from build123d import *

# Parameters (mm, degrees)
SKETCH3_R = 4
P_L_DEPTH = 10


with BuildPart() as part:
    # Sketch1 → Revolve1 (revolve)
    with BuildSketch(Plane.XY):
        with BuildLine():
            Line((-25, 2), (14.8, 2))
            Line((14.8, 2), (15, 1.946410162))
            Line((15, 1.946410162), (15, 1.85))
            ThreePointArc((15, 1.85), (15.029289322, 1.779289322), (15.1, 1.75))
            Line((15.1, 1.75), (15.208578644, 1.75))
            ThreePointArc((15.208578644, 1.75), (15.246846987, 1.757612047), (15.279289322, 1.779289322))
            Line((15.279289322, 1.779289322), (15.5, 2))
            Line((15.5, 2), (26.5, 2))
            Line((26.5, 2), (27, 1.5))
            Line((27, 1.5), (27, 0))
            Line((27, 0), (-27, 0))
            Line((-27, 0), (-27, 4))
            Line((-27, 4), (-25, 4))
            Line((-25, 4), (-25, 2))
        make_face()
    revolve(axis=Axis((0, 0, 0), (1, 0, 0)))

    # Sketch3 → P-L (add)
    with BuildSketch(Plane.ZY.offset(27)):
        Circle(SKETCH3_R)
    extrude(amount=P_L_DEPTH)


solid = part.part
Design review of the part built by this model. Coordinates are the model's own, in mm. A direction names the side the tool comes from. Coordinates: 2 decimals unless noted, no trailing zeros. Order: outer loops, then holes, each group sorted by start corner. A loop starts at its lowest first (then second) coordinate and runs counter-clockwise, first axis right, second up. Notation, with made-up numbers: (26, -11) -> (52, -11) arc R24 cw to (52, 1) -> close; hole circle Ø5 at (84, 9.5). An arc over 180 degrees is marked (long way). Use one line per item in the form item = value. Start each with the question number.
(1) Add section A-A on z = 0. State the section outline as (x, y) points.
(2) Insertion check: pin 1 (3 mm diameter, centred on x = -26, y = 3, fed in from +Z); pin 2 (1 mm diameter, centred on x = -30.5, y = 2, fed in from -Z); pin 3 (1.5 mm diameter, centred on y = 2.5, z = -3, fed in from +X). Each pin has a flat end and moves straight along its axis. Give the tip position at first contact, or say it passes through.
(3) For faces 1 (the flat face through (-25, -2, -1)), 2 (the flat face through (-37, 0, 0)), list the 3-axis set-ups (+Z, -Z, +X, -X, +Y, -Y) from which the entire face can be reached by the end or side of a thin tool; tool diameter is ignored.
(4) Add section C-C on x = 11. State the section outline as (y, z) points, plus the area to 3 significant figures.
(5) For probe 1 along X at (y, z) = (-3.5, -1.5); probe 2 along Y at (x, z) = (-34, -3.5); probe 3 along Y at (x, z) = (-29.5, -0.25), list the stretches that pass through material, from the lowest coordinate up.
Answer block:
q1.outline = (-37, -4) -> (-25, -4) -> (-25, -2) -> (14.8, -2) -> (15, -1.95) -> (15, -1.85) arc R0.1 cw to (15.1, -1.75) -> (15.21, -1.75) arc R0.1 cw to (15.28, -1.78) -> (15.5, -2) -> (26.5, -2) -> (27, -1.5) -> (27, 1.5) -> (26.5, 2) -> (15.5, 2) -> (15.28, 1.78) arc R0.1 cw to (15.21, 1.75) -> (15.1, 1.75) arc R0.1 cw to (15, 1.85) -> (15, 1.95) -> (14.8, 2) -> (-25, 2) -> (-25, 4) -> (-37, 4) -> close
q2.pin_1 = 3.71
q2.pin_2 = -3.71
q2.pin_3 = -25
q3.face_1 = +X
q3.face_2 = +Z, -Z, -X, +Y, -Y
q4.outline = circle Ø4 at (0, 0)
q4.area = 12.6 mm²
q5.probe_1 = -37 to -25
q5.probe_2 = -1.94 to 1.94
q5.probe_3 = -3.99 to 3.99
